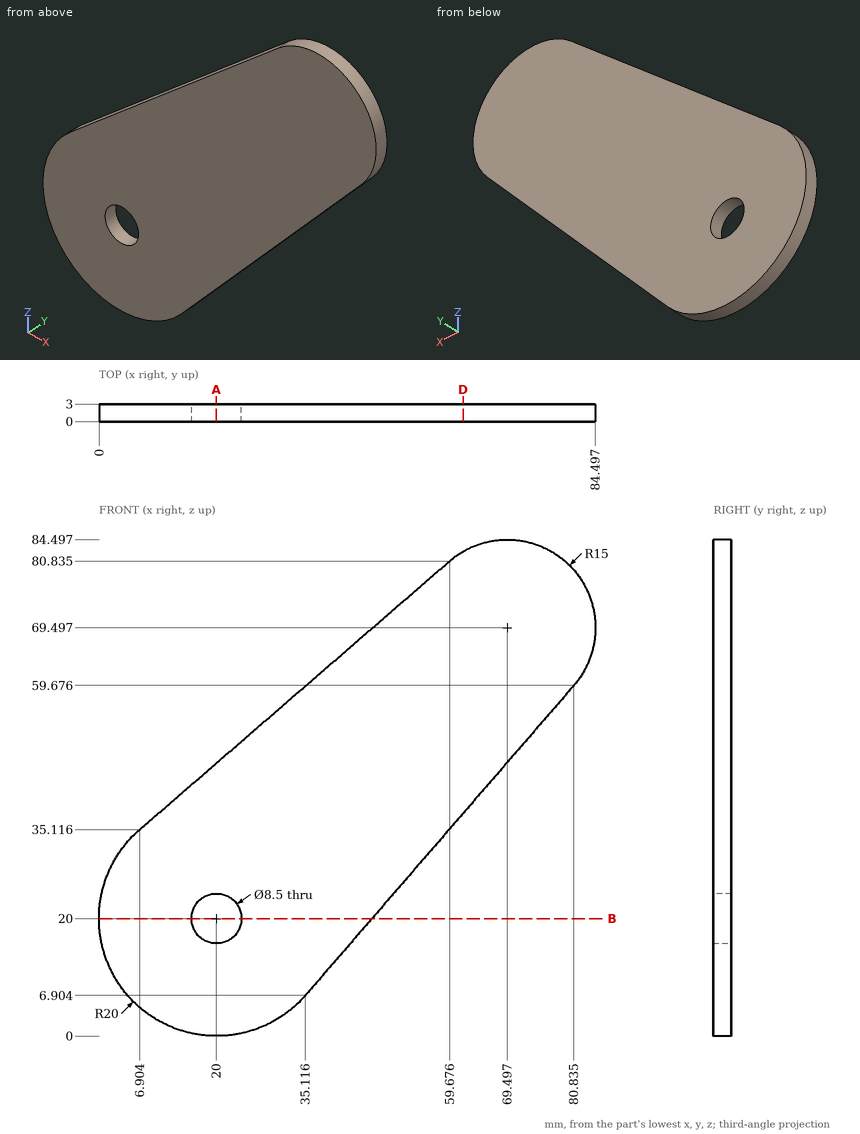
Geometry: see drawing. Coordinates: mm, zero at the bounding-box minimum. Coordinates: 2 decimals unless noted, no trailing zeros. Loops run counter-clockwise (first coordinate to the right, second up) from the corner with the lowest first, then second, coordinate; pieces in that order, holes last. Notation, with made-up numbers: (-38, 27.25) -> (-12, 27.25) arc R18 cw to (-12, 58.25) -> close; hole circle Ø5 at (58, -35.5). An arc over 180 degrees is marked (long way). Use a Markdown table: item, result.
1) Cut plane B-B (z = 20). Return the cut outline in (x, y).
Results found:
| item | result |
|---|---|
| outline | (0, 0) -> (15.75, 0) -> (15.75, 3) -> (0, 3) -> close; (24.25, 0) -> (46.46, 0) -> (46.46, 3) -> (24.25, 3) -> close |
2) Material intervals for line 1 along X through (y, z) = (1.3, 20); line 2 along X through (y, z) = (0.5, 45) (1 decimal); line 3 along X through (y, z) = (1.3, 62) (1 decimal), sorted ascending. Write a range as from..to.
Results found:
| item | result |
|---|---|
| line 1 | x = 0..15.75, 24.25..46.46 |
| line 2 | x = 18.3..68.1 |
| line 3 | x = 37.9..82.5 |
3) Contact query for flat-ended pins moving along their axis: pin 1 (1 mm diameter, centred on x = 15.5, y = 2.5, fed in from -Z); pin 2 (1 mm diameter, centred on y = 1.5, z = 31.5, fed in from +X); pin 3 (1 mm diameter, centred on x = 26, y = 1.5, fed in from -Z). Output: stop coordinate, or through.
Results found:
| item | result |
|---|---|
| pin 1 | stops at z = 0.4 |
| pin 2 | stops at x = 56.86 |
| pin 3 | stops at z = 0.77 |
4) Cut plane D-D (x = 62). Return the cut outline in (y, z) (1 decimal).
Results found:
| item | result |
|---|---|
| outline | (0, 37.9) -> (3, 37.9) -> (3, 82.5) -> (0, 82.5) -> close |
5) Cut plane A-A (x = 20). Return the cut outline in (y, z).
Results found:
| item | result |
|---|---|
| outline | (0, 0) -> (3, 0) -> (3, 15.75) -> (0, 15.75) -> close; (0, 24.25) -> (3, 24.25) -> (3, 46.46) -> (0, 46.46) -> close |
